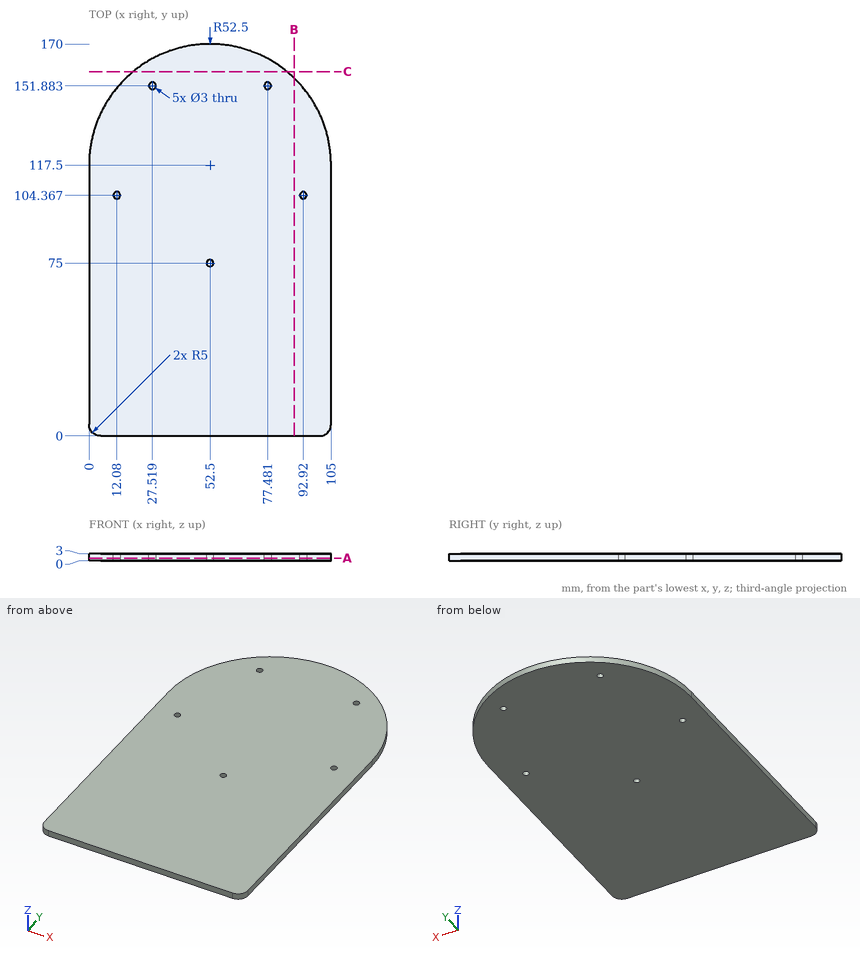
Design review of the part shown in the three views and the two pictorial views. Dimensions are in mm from the part's minimum x, y and z. Coordinates: 2 decimals unless noted, no trailing zeros. Loops run counter-clockwise (first coordinate to the right, second up) from the corner with the lowest first, then second, coordinate; pieces in that order, holes last. Notation, with made-up numbers: M -29,40.25 L 0,40.25 A15 cw 0,52.25 Z; hole C 10.25,-33 d1. An arc over 180 degrees is marked long. Put each result on its own line as item: value. Start each with the question number.
Q1. Add section C-C (y = 158). Write out the cut boundary in (x, z).
Q2. Add section A-A (z = 1.15). Write out the cut boundary in (x, y), and give its area (3 significant figures).
Q3. Clearance check with a flat-ended pin moving along its axis: pin 1 (12 mm diameter, centred on x = 93, y = 46.5, fed in from -Z). State where the tip first meets the part, or that it passes through.
Q4. Wall thickness on line 1 (X direction, y = 75, z = 2.3); line 2 (Y direction, x = 12, z = 1.75) (1 decimal); line 3 (Y direction, x = 73.5, z = 2.9): over which ranges is each line inside the solid? List them lowest first.
Q5. Add section B-B (x = 89). Write out the cut boundary in (y, z), and give its area (3 significant figures).
Answers:
1. outline: M 19.09,0 L 85.91,0 L 85.91,3 L 19.09,3 Z
2. outline: M 0,5 A5 ccw 5,0 L 100,0 A5 ccw 105,5 L 105,117.5 A52.5 ccw 0,117.5 Z; hole C 12.08,104.37 d3; hole C 27.52,151.88 d3; hole C 52.5,75 d3; hole C 77.48,151.88 d3; hole C 92.92,104.37 d3
2. area: 16,600 mm^2
3. pin 1: stops at z = 0
4. line 1: x = 0 to 51, 54 to 105
4. line 2: y = 0 to 102.9, 105.9 to 150.9
4. line 3: y = 0 to 165.62
5. outline: M 0,0 L 155.24,0 L 155.24,3 L 0,3 Z
5. area: 466 mm^2
